The figure shows three views and two pictorial views of one solid part (mm, origin at its lowest corner). Answer the questions. A direction names the side the tool comes from. Coordinates: 2 decimals unless noted, no trailing zeros. Write each loop counter-clockwise with the first axis right and the second up, starting at its lowest first coordinate (ties: lowest second). Pieces come first, ordered by that corner, then holes.
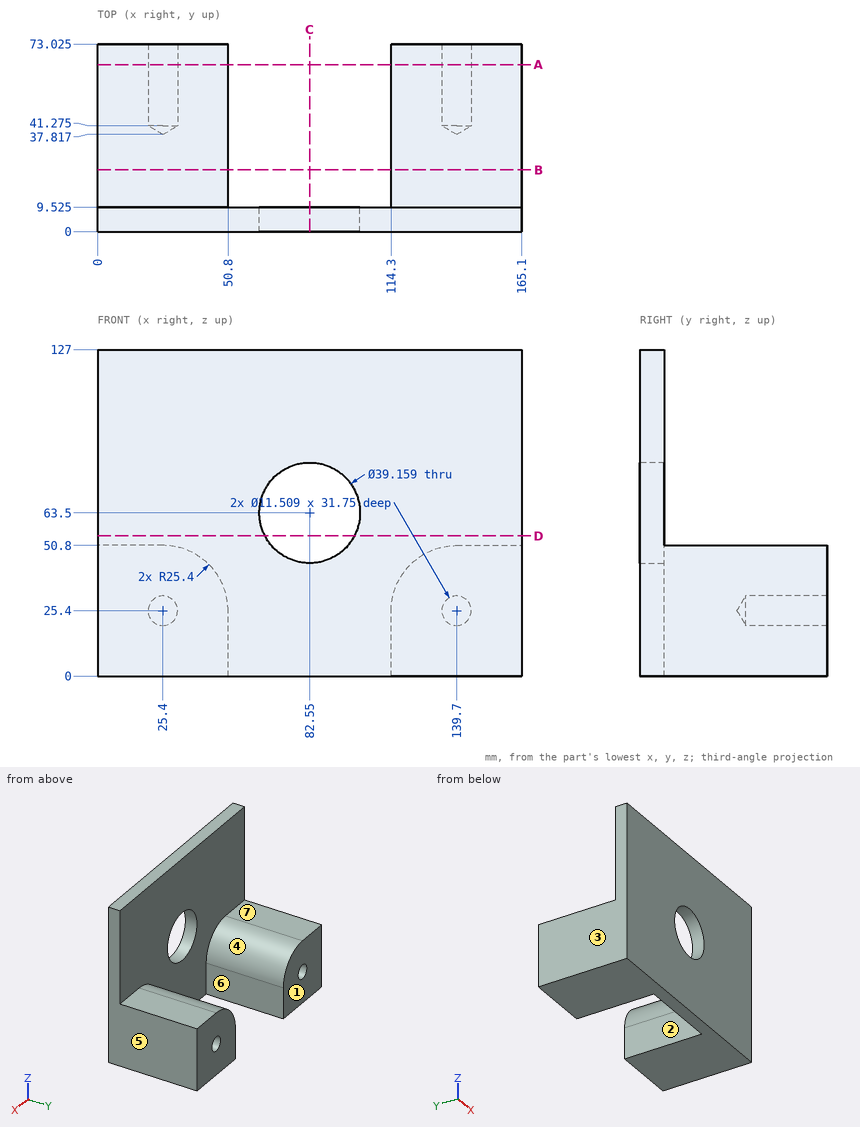
Item 1: Given pin 1 (20.5 mm diameter, centred on x = 150, y = 26, fed in from +Z); pin 2 (9 mm diameter, centred on x = 139.7, z = 25.4, fed in from +Y); pin 3 (5 mm diameter, centred on x = 78.5, z = 102, fed in from +Y) (3 decimals), each flat-ended and moving along its own axis, determine where each tip first touches the part or whether it passes through.
Item 2: The part is cut by section B-B (y = 24). Give the vertices of the cut face in (x, z).
Item 3: The part is cut by section A-A (y = 65). Give the vertices of the cut face in (x, z) (1 decimal).
Item 4: Find the intervals of material crossed by probe 1 along X at (y, z) = (63, 25); probe 2 along Z at (x, y) = (25, 60); probe 3 along X at (y, z) = (40.5, 14), in increasing order.
Item 5: For the marked faces 4, 5, 6 and 7, determine the directions among +Z, -Z, +X, -X, +Y, -Y from which every point of the face is accessible in a straight line to the end or side of a thin tool.
Item 6: The part is cut by section C-C (x = 82.55). Give the vertices of the cut face in (y, z) (1 decimal).
Item 7: The part is cut by section D-D (z = 54.5). Give the vertices of the cut face in (x, y) (1 decimal), and give its area (3 significant figures).
Item 8: Determine the mould class of the marked faces 1, 2 and 3 for opening direction X: +X half, -X half, draft (parallel to the pull), parting line (faces both ways), or undercut.
Answer:
1. pin 1: stops at z = 50.8
1. pin 2: stops at y = 40.52
1. pin 3: stops at y = 9.525
2. outline: (0, 0) - (50.8, 0) - (50.8, 25.4) arc R25.4 ccw to (25.4, 50.8) - (0, 50.8) - close; (114.3, 0) - (165.1, 0) - (165.1, 50.8) - (139.7, 50.8) arc R25.4 ccw to (114.3, 25.4) - close
3. outline: (0, 0) - (50.8, 0) - (50.8, 25.4) arc R25.4 ccw to (25.4, 50.8) - (0, 50.8) - close; (114.3, 0) - (165.1, 0) - (165.1, 50.8) - (139.7, 50.8) arc R25.4 ccw to (114.3, 25.4) - close; hole circle Ø11.5 at (25.4, 25.4); hole circle Ø11.5 at (139.7, 25.4)
4. probe 1: x = 0 to 19.66, 31.14 to 50.8, 114.3 to 133.96, 145.44 to 165.1
4. probe 2: z = 0 to 19.66, 31.14 to 50.8
4. probe 3: x = 0 to 50.8, 114.3 to 165.1
5. face 4: +Z, +Y
5. face 5: +Z, -Z, +X, +Y, -Y
5. face 6: +Z, -Z, +Y
5. face 7: +Z, +X, -X, +Y
6. outline: (0, 0) - (9.5, 0) - (9.5, 43.9) - (0, 43.9) - close; (0, 83.1) - (9.5, 83.1) - (9.5, 127) - (0, 127) - close
7. outline: (0, 0) - (65.2, 0) - (65.2, 9.5) - (0, 9.5) - close; (99.9, 0) - (165.1, 0) - (165.1, 9.5) - (99.9, 9.5) - close
7. area: 1,240 mm2
8. face 1: draft
8. face 2: undercut
8. face 3: -X half
